Source: CAD feature listing. Evaluate the final solid. Frame: model axes, mm. Face numbers are marked on the shaded views. A direction names the side the tool comes from. Give positions to 0.01 mm unless a question says otherwise; leave off trailing zeros. Write each loop counter-clockwise with the first axis right and the second up, starting at its lowest first coordinate (ties: lowest second). Pieces come first, ordered by that corner, then holes. Notation, with made-up numbers: (-19, 35) -> (-15, 35) arc R28 ccw to (-15, 70) -> close; hole circle Ø11 at (54.5, -14). An arc over 180 degrees is marked (long way). Use one line per item in the form item = value. Start each with the question number.
(1) Cut plane A-A, the plane z = 0. Output: boundary loops of the cut face in (x, y).
(2) Cut plane D-D, the plane y = 2.95. Output: boundary loops of the cut face in (x, z).
(3) First-contact query: P1, Ø1.5, axis at y = 3.5, z = 4, coming from the +X side. Flat tip, straight axial feed; report the tip coordinate or a pass-through.
(4) Material intervals for line 1 along X through (y, z) = (3.8, 0); line 2 along X through (y, z) = (0.1, 0); line 3 along X through (y, z) = (1.55, 0), sorted ascending. Write a range as from..to.
(5) Draft query along Z for the marked faces 1, 2 and 3. Return one class per face: pulls with the +Z half, pulls with the -Z half, needs draft (parallel to the pull), parting line crosses it, or undercut.
(6) Set-up query: the marked faces 4, 5 and 6. Return all of +Z, -Z, +X, -X, +Y, -Y with unobstructed straight access to the full face (end or side cutting, diameter ignored); none if empty.
(7) Cut plane B-B, the plane x = 0. Output: boundary loops of the cut face in (y, z).
(8) Cut plane C-C, the plane z = 3. Output: boundary loops of the cut face in (x, y).
from build123d import *

# Parameters (mm, degrees)
SKETCH1_R           = 4
SKETCH1_R_2         = 1.5
BOSS_EXTRUDE1_DEPTH = 4
SKETCH2_R           = 3.25
SKETCH2_R_2         = 1.75
CUT_EXTRUDE1_DEPTH  = 0.25
BOSS_EXTRUDE2_START = -0.9
SKETCH3_R           = 4.75
SKETCH3_R_2         = 4
BOSS_EXTRUDE2_DEPTH = 0.9


with BuildPart() as part:
    # Sketch1 → Boss-Extrude1 (new body)
    with BuildSketch(Plane(origin=(0, 0, 0), x_dir=(1, 0, 0), z_dir=(0, 1, 0))):
        with Locations(Location((0, 0, 0), (0, 0, 270))):
            Circle(SKETCH1_R)
        with Locations(Location((0, 0, 0), (0, 0, 270))):
            Circle(SKETCH1_R_2, mode=Mode.SUBTRACT)
    extrude(amount=BOSS_EXTRUDE1_DEPTH)

    # Sketch2 → Cut-Extrude1 (cut)
    with BuildSketch(Plane(origin=(0, 4, 0), x_dir=(1, 0, 0), z_dir=(0, 1, 0))):
        with Locations(Location((0, 0, 0), (0, 0, 270))):
            Circle(SKETCH2_R)
        with Locations(Location((0, 0, 0), (0, 0, 270))):
            Circle(SKETCH2_R_2, mode=Mode.SUBTRACT)
    cut_extrude1 = extrude(amount=-CUT_EXTRUDE1_DEPTH, mode=Mode.SUBTRACT)

    # Mirror1: Cut-Extrude1 across plane
    add(cut_extrude1.mirror(Plane.ZX.offset(2)), mode=Mode.SUBTRACT)

    # Sketch3 → Boss-Extrude2 (add)
    with BuildSketch(Plane(origin=(0, 4, 0), x_dir=(1, 0, 0), z_dir=(0, 1, 0)).offset(BOSS_EXTRUDE2_START)):
        with Locations(Location((0, 0, 0), (0, 0, 270))):
            Circle(SKETCH3_R)
        with Locations(Location((0, 0, 0), (0, 0, 270))):
            Circle(SKETCH3_R_2, mode=Mode.SUBTRACT)
    extrude(amount=BOSS_EXTRUDE2_DEPTH)


solid = part.part
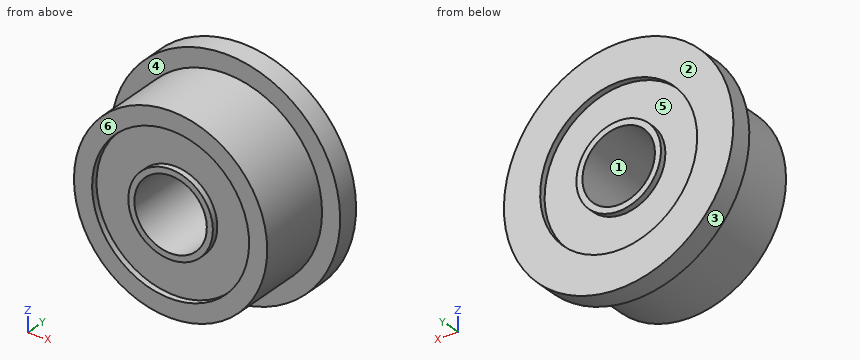
Geometry says:
q1.outline = (-4.75, 3.1) -> (-4, 3.1) -> (-4, 0) -> (-3.25, 0) -> (-3.25, 0.25) -> (-1.75, 0.25) -> (-1.75, 0) -> (-1.5, 0) -> (-1.5, 4) -> (-1.75, 4) -> (-1.75, 3.75) -> (-3.25, 3.75) -> (-3.25, 4) -> (-4.75, 4) -> close; (1.5, 0) -> (1.75, 0) -> (1.75, 0.25) -> (3.25, 0.25) -> (3.25, 0) -> (4, 0) -> (4, 3.1) -> (4.75, 3.1) -> (4.75, 4) -> (3.25, 4) -> (3.25, 3.75) -> (1.75, 3.75) -> (1.75, 4) -> (1.5, 4) -> close
q2.outline = circle Ø8 at (0, 0); hole circle Ø3 at (0, 0)
q3.P1 = 3.46
q4.line_1 = -4.75..-3.25, -1.75..-1.5, 1.5..1.75, 3.25..4.75
q4.line_2 = -4..-3.25, -1.75..-1.5, 1.5..1.75, 3.25..4
q4.line_3 = -4..-1.5, 1.5..4
q5.face_1 = undercut
q5.face_2 = needs draft
q5.face_3 = parting line crosses it
q6.face_4 = -Y
q6.face_5 = +Y
q6.face_6 = +Z, -Z, +X, -X, -Y
q7.outline = (0, -4) -> (3.1, -4) -> (3.1, -4.75) -> (4, -4.75) -> (4, -3.25) -> (3.75, -3.25) -> (3.75, -1.75) -> (4, -1.75) -> (4, -1.5) -> (0, -1.5) -> (0, -1.75) -> (0.25, -1.75) -> (0.25, -3.25) -> (0, -3.25) -> close; (0, 1.5) -> (4, 1.5) -> (4, 1.75) -> (3.75, 1.75) -> (3.75, 3.25) -> (4, 3.25) -> (4, 4.75) -> (3.1, 4.75) -> (3.1, 4) -> (0, 4) -> (0, 3.25) -> (0.25, 3.25) -> (0.25, 1.75) -> (0, 1.75) -> close
q8.outline = (-3.68, 3.1) -> (-2.65, 3.1) -> (-2.65, 0) -> (-1.25, 0) -> (-1.25, 0.25) -> (1.25, 0.25) -> (1.25, 0) -> (2.65, 0) -> (2.65, 3.1) -> (3.68, 3.1) -> (3.68, 4) -> (1.25, 4) -> (1.25, 3.75) -> (-1.25, 3.75) -> (-1.25, 4) -> (-3.68, 4) -> close
